from build123d import *

# Parameters (mm, degrees)
SKETCH1_R           = 2.75
BOSS_EXTRUDE1_DEPTH = 7
FILLET1_R           = 2.7
SKETCH2_R           = 3.061280108
BOSS_EXTRUDE2_DEPTH = 1
BOSS_EXTRUDE3_DEPTH = 0.5
FILLET2_R           = 0.7


with BuildPart() as part:
    # Sketch1 → Boss-Extrude1 (new body)
    with BuildSketch(Plane(origin=(0, 0, 0), x_dir=(1, 0, 0), z_dir=(0, 1, 0))):
        with Locations(Location((0, 0, 0), (0, 0, 270))):
            Circle(SKETCH1_R)
    extrude(amount=BOSS_EXTRUDE1_DEPTH)

    # Fillet1
    fillet1_edges = [part.edges().sort_by_distance(p)[0] for p in [
        (0, 7, -2.75),
    ]]
    fillet(fillet1_edges, radius=FILLET1_R)

    # Sketch2 → Boss-Extrude2 (add)
    with BuildSketch(Plane.XZ):
        with Locations(Location((0, 0, 0), (0, 0, 270))):
            Circle(SKETCH2_R)
    extrude(amount=BOSS_EXTRUDE2_DEPTH)

    # Sketch3 → Boss-Extrude3 (add)
    with BuildSketch(Plane.XZ.offset(1)):
        with BuildLine():
            ThreePointArc((-2.522635735, 1.734285112), (-2.648517192, 1.535184868), (-2.758717126, 1.326994996))
            Line((-2.758717126, 1.326994996), (0, 1.326994996))
            Line((0, 1.326994996), (0, 1.734285112))
            Line((0, 1.734285112), (-2.522635735, 1.734285112))
        make_face()
        with BuildLine():
            Line((-13.203045703, 1.326994996), (-2.758717126, 1.326994996))
            ThreePointArc((-2.758717126, 1.326994996), (-2.648517192, 1.535184868), (-2.522635735, 1.734285112))
            Line((-2.522635735, 1.734285112), (-13.203045703, 1.734285112))
            Line((-13.203045703, 1.734285112), (-13.203045703, 1.326994996))
        make_face()
        with BuildLine():
            Line((-2.522635735, -1.734285112), (0, -1.734285112))
            Line((0, -1.734285112), (0, -1.326994996))
            Line((0, -1.326994996), (-2.758717126, -1.326994996))
            ThreePointArc((-2.758717126, -1.326994996), (-2.648517192, -1.535184868), (-2.522635735, -1.734285112))
        make_face()
        with BuildLine():
            Line((-13.203045703, -1.734285112), (-2.522635735, -1.734285112))
            ThreePointArc((-2.522635735, -1.734285112), (-2.648517192, -1.535184868), (-2.758717126, -1.326994996))
            Line((-2.758717126, -1.326994996), (-13.203045703, -1.326994996))
            Line((-13.203045703, -1.326994996), (-13.203045703, -1.734285112))
        make_face()
    extrude(amount=BOSS_EXTRUDE3_DEPTH)

    # Fillet2
    # the kernel refuses this fillet: 0.7 mm, written as the material it takes off along each edge
    with BuildSketch(Plane(origin=(0, -1.5, -3.411336095), x_dir=(0, 1, 0), z_dir=(0, 0, 1)), Plane(origin=(0, -1.5, -0.350055987), x_dir=(0, 1, 0), z_dir=(0, 0, 1))) as fillet2_piece_1:
        with BuildLine():
            CenterArc((0.7, 0.670820393), FILLET2_R, 180, 73.398450401)
            Line((0, 0.670820393), (-0.014, 0.670820393))
            Line((-0.014, 0.670820393), (-0.014, 0))
            Line((-0.014, 0), (0, -0.014))
            ThreePointArc((0, -0.014), (0.25, -0.014), (0.496, -0.013416408))
            Line((0.496, -0.013416408), (0.5, 0))
        make_face()
    extrude(amount=3.761392082, mode=Mode.SUBTRACT)


solid = part.part
The model under review builds one solid part; all positions refer to its coordinate system, in mm. Round coordinates to 2 decimals unless told otherwise and drop trailing zeros. Write each loop counter-clockwise with the first axis right and the second up, starting at its lowest first coordinate (ties: lowest second). Pieces come first, ordered by that corner, then holes. Notation, with made-up numbers: (-15, 33) - (39, 33) arc R21 cw to (39, 49) - close; hole circle Ø7 at (74.5, 13). An arc over 180 degrees is marked (long way). One line per item, written item: value. Start each with the question number.
1. To check wall thickness, follow L1, parallel to X at y = 1.25, z = 0; L2, parallel to Y at x = 1.25, z = 1.25; L3, parallel to Y at x = -1.5, z = -1.25. State the ranges of each line that lie inside material, in increasing order. Write a range as from..to.
2. Consider section B-B on y = 3.5. Write out the cut boundary in (x, z).
3. Clearance check with flat-ended pins moving along their axes: P1, Ø1.5, axis at y = 1, z = 0, coming from the +X side; P2, Ø1, axis at y = 2, z = -1.5, coming from the -X side; P3, Ø1, axis at y = 2, z = 1.5, coming from the +X side; P4, Ø1.5, axis at x = -6.5, y = 1.5, coming from the +Z side. State where each tip first meets the part, or that it passes through.
4. Consider section A-A on x = -5.5. Write out the cut boundary in (y, z), and give its area (3 significant figures).
Checks:
1. L1: x = -2.75..2.75
1. L2: y = -1..6.38
1. L3: y = -1..6.22
2. outline: circle Ø5.5 at (0, 0)
3. P1: stops at x = 2.75
3. P2: stops at x = -2.56
3. P3: stops at x = 2.56
3. P4: passes through
4. outline: (-1.5, -1.73) - (-1, -1.73) - (-1, -1.33) - (-1.5, -1.33) - close; (-1.5, 1.33) - (-1, 1.33) - (-1, 1.73) - (-1.5, 1.73) - close
4. area: 0.407 mm^2
